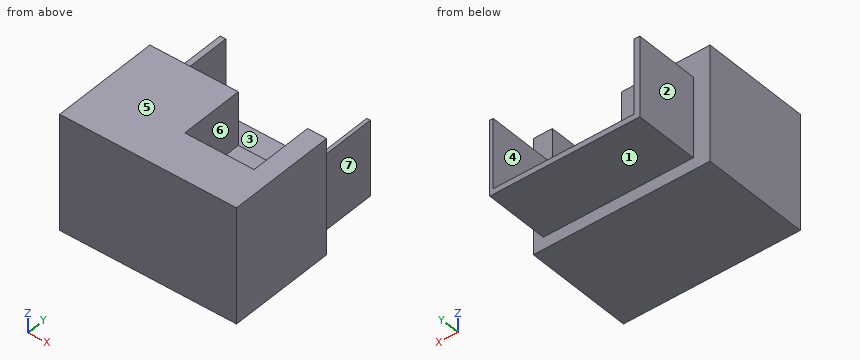
Autodesk Inventor part; units mm, degrees
ref_plane "YZ Plane" through (0, 0, 0) normal (1, 0, 0) x (0, 1, 0)
ref_plane "XZ Plane" through (0, 0, 0) normal (0, 1, 0) x (-1, 0, 0)
ref_plane "XY Plane" through (0, 0, 0) normal (0, 0, 1) x (1, 0, 0)
sketch "스케치1" plane through (0, 0, 0) normal (0, 0, 1) x (1, 0, 0)
  line L0 (68.5732, -42.1218) -> (-68.5732, -42.1218)
  line L1 (-68.5732, -42.1218) -> (-68.5732, 42.1218)
  line L2 (-68.5732, 42.1218) -> (68.5732, 42.1218)
  line L3 (68.5732, 42.1218) -> (68.5732, -42.1218)
  line L4 (68.5732, -42.1218) -> (-68.5732, 42.1218) construction
  line L5 (-68.5732, -42.1218) -> (68.5732, 42.1218) construction
  point P0 (0, 0)
extrude "돌출1" add sketch "스케치1" along normal blind 90
sketch "스케치2" plane through (-68.5732, 42.1218, 0) normal (0, 1, 0) x (1, 0, 0)
  line L0 (0, -90) -> (137.1464, -90)
  line L1 (68.5732, -90) -> (122.3358, -90)
  line L2 (122.3358, -90) -> (122.3358, -48.4921)
  line L3 (122.3358, -48.4921) -> (68.5732, -48.4921)
  line L4 (68.5732, -48.4921) -> (68.5732, -90)
  point P0 (68.5732, 0)
extrude "돌출2" cut sketch "스케치2" against normal blind 50
sketch "스케치3" plane through (-68.5732, 42.1218, 0) normal (0, 1, 0) x (1, 0, 0)
  line L0 (13.0375, -71.9969) -> (13.0375, -9.4777)
  line L1 (13.0375, -9.4777) -> (129.4297, -9.4777)
  line L2 (129.4297, -9.4777) -> (129.4297, -68.3389)
  line L3 (129.4297, -68.3389) -> (126.7693, -68.3389)
  line L4 (126.7693, -68.3389) -> (126.7693, -13.8008)
  line L5 (126.7693, -13.8008) -> (17.3606, -13.8008)
  line L6 (17.3606, -13.8008) -> (17.3606, -71.9969)
  line L7 (17.3606, -71.9969) -> (13.0375, -71.9969)
  point P0 (68.5732, 0)
extrude "돌출3" add sketch "스케치3" along normal blind 50
properties part number "240503_3Dsketch02"
CAD build for the part. Positions are in the model's coordinates, mm. Face numbers are marked on the shaded views. A direction names the side the tool comes from. Round coordinates to 2 decimals unless told otherwise and drop trailing zeros. Write each loop counter-clockwise with the first axis right and the second up, starting at its lowest first coordinate (ties: lowest second). Pieces come first, ordered by that corner, then holes. Notation, with made-up numbers: M 7.5,85 L 46.5,85 A22 cw 46.5,107 Z; hole C 88.25,-23.5 d8. An arc over 180 degrees is marked long. One line per question, with ' | ' between items.
1. Probe L1, parallel to X at y = 8, z = 77.5; L2, parallel to X at y = 73.5, z = 49; L3, parallel to Y at x = 4, z = 21.5. List the from-to ranges inside material, lowest first. Write a range as from..to.
Working result:
L1: -68.57..0, 53.76..68.57 | L2: -55.54..-51.21, 58.2..60.86 | L3: -42.12..42.12
2. Pin check, flat tips, straight feed: pin 1 Ø2 at (x, z) = (-45, 64.5) entering from +Y; pin 2 Ø6 at (y, z) = (52, 31) entering from -X; pin 3 Ø2 at (x, y) = (-54.5, 58.5) entering from +Z. Stop position of each tip, or through.
Working result:
pin 1: y = 42.12 | pin 2: x = -55.54 | pin 3: z = 72
3. Cut at A-A on x = 4.5. Write the cut outline in (y, z).
Working result:
outline: M -42.12,0 L 42.12,0 L 42.12,9.48 L 92.12,9.48 L 92.12,13.8 L 42.12,13.8 L 42.12,48.49 L -7.88,48.49 L -7.88,90 L -42.12,90 Z
4. Mould opens along X. For the marked faces 4, 5, 6 and 7 say: pulls with the +X half, pulls with the -X half, needs draft (parallel to the pull), parting line crosses it, or undercut.
Working result:
face 4: undercut | face 5: needs draft | face 6: undercut | face 7: pulls with the +X half
5. Cut at B-B on z = 78. Write the cut outline in (x, y).
Working result:
outline: M -68.57,-42.12 L 68.57,-42.12 L 68.57,42.12 L 53.76,42.12 L 53.76,-7.88 L 0,-7.88 L 0,42.12 L -68.57,42.12 Z
6. Cut at C-C on y = 1. Write the cut outline in (x, z).
Working result:
outline: M -68.57,0 L 68.57,0 L 68.57,90 L 53.76,90 L 53.76,48.49 L 0,48.49 L 0,90 L -68.57,90 Z
7. Cut at D-D on z = 45. Write the cut outline in (x, y), and give its area (3 significant figures).
Working result:
outline: M -68.57,-42.12 L 68.57,-42.12 L 68.57,42.12 L 60.86,42.12 L 60.86,92.12 L 58.2,92.12 L 58.2,42.12 L -51.21,42.12 L -51.21,92.12 L -55.54,92.12 L -55.54,42.12 L -68.57,42.12 Z | area: 11,900 mm2
8. Which spindle directions (+Z, -Z, +X, -X, +Y, -Y) get a long thin tool onto all of the face, cutting with end or side? Do the marked faces 1, 2 and 3. Say none if no direction does.
Working result:
face 1: -Z, +X, -X, +Y | face 2: +Z, -Z, -X, +Y | face 3: +Z, +Y
